Could you check a few things on this drawing? It's one solid part, dimensions in mm from its lowest x, y, z. A direction names the side the tool comes from. Round coordinates to 2 decimals unless told otherwise and drop trailing zeros. Loops run counter-clockwise (first coordinate to the right, second up) from the corner with the lowest first, then second, coordinate; pieces in that order, holes last. Notation, with made-up numbers: (73, -32) -> (114, -32) arc R7 cw to (114, -26) -> close; hole circle Ø3 at (16.25, 65). An arc over 180 degrees is marked (long way). Put each result on its own line as item: value. Start each with the question number.
1. Which directions (+Z, -Z, +X, -X, +Y, -Y) give clear straight access to the entire face, cutting with the end or side of a thin tool? Please do the marked faces 1 and 2.
2. Imagine slicing it at A-A, the plane x = 19.05. Please give me the cut outline in (y, z) (1 decimal), and give its area (3 significant figures).
3. I need wall thicknesses on line 1 (Y direction, x = 19.05, z = 4.5) (1 decimal); line 2 (Z direction, x = 5.08, y = 3.75); line 3 (X direction, y = 13.5, z = 5.25) (1 decimal). Which ranges of each line are inside material? Lowest first, please. Write a range as [from, to].
4. If we mould it in two halves opening along X, with no side actions, what happens to the marked faces 3, 4 and 5? For each: pulls with the +X half, pulls with the -X half, needs draft (parallel to the pull), parting line crosses it, or undercut.
5. Imagine slicing it at C-C, the plane y = 3. Please give me the cut outline in (x, z).
6. Imagine slicing it at B-B, the plane y = 31. Please give me the cut outline in (x, z), and give its area (3 significant figures).
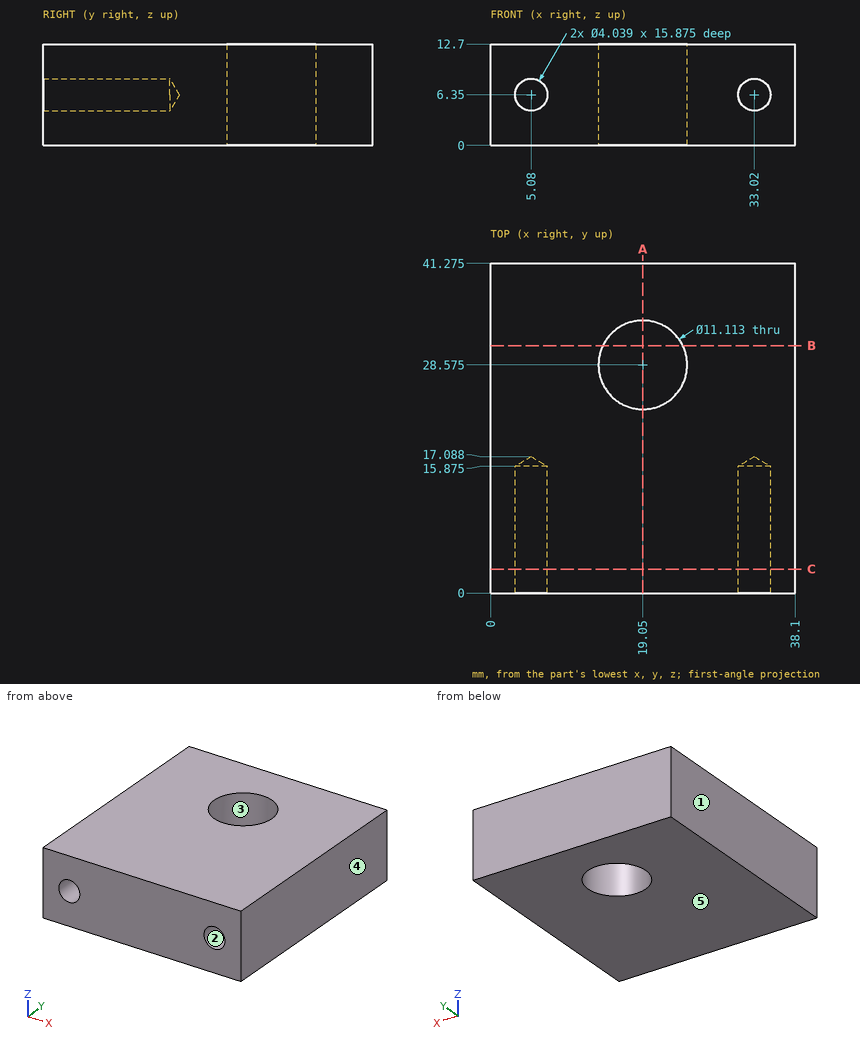
Entries:
1. face 1: +Z, -Z, -X, +Y, -Y
1. face 2: -Y
2. outline: (0, 0) -> (23, 0) -> (23, 12.7) -> (0, 12.7) -> close; (34.1, 0) -> (41.3, 0) -> (41.3, 12.7) -> (34.1, 12.7) -> close
2. area: 383 mm^2
3. line 1: [0, 23], [34.1, 41.3]
3. line 2: [0, 4.33], [8.37, 12.7]
3. line 3: [0, 3.4], [6.8, 31.3], [34.7, 38.1]
4. face 3: undercut
4. face 4: pulls with the +X half
4. face 5: needs draft
5. outline: (0, 0) -> (38.1, 0) -> (38.1, 12.7) -> (0, 12.7) -> close; hole circle Ø4.04 at (5.08, 6.35); hole circle Ø4.04 at (33.02, 6.35)
6. outline: (0, 0) -> (14.05, 0) -> (14.05, 12.7) -> (0, 12.7) -> close; (24.05, 0) -> (38.1, 0) -> (38.1, 12.7) -> (24.05, 12.7) -> close
6. area: 357 mm^2
